from build123d import *

# Parameters (mm, degrees)
SKETCH1_W               = 6
SKETCH1_H               = 15
SKETCH1_W_2             = 8
SKETCH1_H_2             = 28.7
BOSS_EXTRUDE1_DEPTH     = 9
SKETCH2_R               = 2.65
CUT_EXTRUDE1_DEPTH      = 34.176648414
SKETCH5_W               = 10
SKETCH5_H               = 5.3
BOSS_EXTRUDE4_DEPTH     = 5
SKETCH6_W               = 12
SKETCH6_H               = 5.3
BOSS_EXTRUDE5_DEPTH     = 2
SKETCH7_W               = 14
SKETCH7_H               = 6.2
CUT_EXTRUDE2_DEPTH      = 1.2
SKETCH8_R               = 1.45
CUT_EXTRUDE3_DEPTH      = 8
CUT_EXTRUDE4_DEPTH      = 36.716802768
CUT_EXTRUDE4_DEPTH_BACK = 36.716802768
SKETCH9_R               = 1.75
FILLET1_R               = 5
FILLET2_R               = 6
FILLET3_R               = 3


# Some blends are built 0.0001 mm under size
with BuildPart() as part:
    # Sketch1 → Boss-Extrude1 (new, symmetric)
    with BuildSketch(Plane.XY):
        with Locations((11, -7.5)):
            Rectangle(SKETCH1_W, SKETCH1_H)
        with Locations((4, -14.35)):
            Rectangle(SKETCH1_W_2, SKETCH1_H_2)
    extrude(amount=BOSS_EXTRUDE1_DEPTH, both=True)

    # Sketch2 → Cut-Extrude1 (cut, through all)
    with BuildSketch(Plane(origin=(14, 0, 0), x_dir=(0, 0, -1), z_dir=(1, 0, 0))):
        with Locations(Location((5, -4.2, 0), (0, 0, 90))):
            Circle(SKETCH2_R)
        with Locations(Location((-5, -4.2, 0), (0, 0, 90))):
            Circle(SKETCH2_R)
    extrude(amount=-CUT_EXTRUDE1_DEPTH, mode=Mode.SUBTRACT)

    # Sketch5 → Boss-Extrude4 (add)
    with BuildSketch(Plane.XY.offset(9)):
        with Locations((5, -4.2)):
            Rectangle(SKETCH5_W, SKETCH5_H)
    boss_extrude4 = extrude(amount=BOSS_EXTRUDE4_DEPTH)

    # Sketch6 → Boss-Extrude5 (add)
    with BuildSketch(Plane.XY.offset(14)):
        with Locations((6, -4.2)):
            Rectangle(SKETCH6_W, SKETCH6_H)
    boss_extrude5 = extrude(amount=BOSS_EXTRUDE5_DEPTH)

    # Mirror2: Boss-Extrude4, Boss-Extrude5 across plane
    add(boss_extrude4.mirror(Plane.XY))
    add(boss_extrude5.mirror(Plane.XY))

    # Sketch7 → Cut-Extrude2 (cut)
    with BuildSketch(Plane(origin=(0, 0, 0), x_dir=(1, 0, 0), z_dir=(0, 1, 0))):
        with Locations((7, 0)):
            Rectangle(SKETCH7_W, SKETCH7_H)
    extrude(amount=-CUT_EXTRUDE2_DEPTH, mode=Mode.SUBTRACT)

    # Sketch8 → Cut-Extrude3 (cut)
    with BuildSketch(Plane(origin=(0, -1.2, 0), x_dir=(1, 0, 0), z_dir=(0, 1, 0))):
        with Locations(Location((7, 0, 0), (0, 0, 270))):
            Circle(SKETCH8_R)
    extrude(amount=-CUT_EXTRUDE3_DEPTH, mode=Mode.SUBTRACT)

    # Sketch9 → Cut-Extrude4 (cut, two sides: drawn at the far end of the back side and taken through both)
    with BuildSketch(Plane.ZY.offset(-CUT_EXTRUDE4_DEPTH_BACK)):
        with Locations(Location((0, -18.7, 0), (0, 0, 90))):
            Circle(SKETCH9_R)
    extrude(amount=CUT_EXTRUDE4_DEPTH + CUT_EXTRUDE4_DEPTH_BACK, mode=Mode.SUBTRACT)

    # Fillet1
    fillet1_edges = [part.edges().sort_by_distance(p)[0] for p in [
        (8, -28.7, 0),
    ]]
    fillet(fillet1_edges, radius=FILLET1_R)

    # Fillet2
    fillet2_edges = [part.edges().sort_by_distance(p)[0] for p in [
        (14, -15, 0),
    ]]
    fillet(fillet2_edges, radius=FILLET2_R - 0.0001)  # a hair under: the kernel refuses the full size

    # Fillet3
    # the kernel refuses this fillet: 3 mm, written as the material it adds along each edge
    with BuildSketch(Plane(origin=(10, -6.85, 9), x_dir=(0, -1, 0), z_dir=(-1, 0, 0))) as fillet3_piece_1:
        with BuildLine():
            CenterArc((FILLET3_R, FILLET3_R), FILLET3_R, 180, 90)
            Line((0, FILLET3_R), (-FILLET3_R * 0.02, FILLET3_R))
            Line((-FILLET3_R * 0.02, FILLET3_R), (-FILLET3_R * 0.02, -FILLET3_R * 0.02))
            Line((-FILLET3_R * 0.02, -FILLET3_R * 0.02), (FILLET3_R, -FILLET3_R * 0.02))
            Line((FILLET3_R, -FILLET3_R * 0.02), (FILLET3_R, 0))
        make_face()
    extrude(amount=10)
    with BuildSketch(Plane(origin=(0, -1.55, 9), x_dir=(0, 1, 0), z_dir=(1, 0, 0))) as fillet3_piece_2:
        with BuildLine():
            CenterArc((3, 2.626309197), FILLET3_R, 180, 61.09666546)
            Line((0, 2.626309197), (-0.06, 2.626309197))
            Line((-0.06, 2.626309197), (-0.06, 0))
            Line((-0.06, 0), (0, -0.06))
            ThreePointArc((0, -0.06), (0.775, -0.06), (1.521, -0.052526184))
            Line((1.521, -0.052526184), (1.55, 0))
        make_face()
    extrude(amount=10)
    with BuildSketch(Plane(origin=(10, -6.85, -9), x_dir=(0, -1, 0), z_dir=(-1, 0, 0))) as fillet3_piece_3:
        with BuildLine():
            CenterArc((FILLET3_R, -FILLET3_R), FILLET3_R, 90, 90)
            Line((0, -FILLET3_R), (-FILLET3_R * 0.02, -FILLET3_R))
            Line((-FILLET3_R * 0.02, -FILLET3_R), (-FILLET3_R * 0.02, FILLET3_R * 0.02))
            Line((-FILLET3_R * 0.02, FILLET3_R * 0.02), (FILLET3_R, FILLET3_R * 0.02))
            Line((FILLET3_R, FILLET3_R * 0.02), (FILLET3_R, 0))
        make_face()
    extrude(amount=10)
    with BuildSketch(Plane(origin=(0, -1.55, -9), x_dir=(0, 1, 0), z_dir=(1, 0, 0))) as fillet3_piece_4:
        with BuildLine():
            CenterArc((3, -2.626309197), FILLET3_R, 118.90333454, 61.09666546)
            Line((0, -2.626309197), (-0.06, -2.626309197))
            Line((-0.06, -2.626309197), (-0.06, 0))
            Line((-0.06, 0), (0, 0.06))
            ThreePointArc((0, 0.06), (0.775, 0.06), (1.521, 0.052526184))
            Line((1.521, 0.052526184), (1.55, 0))
        make_face()
    extrude(amount=10)


solid = part.part
Geometry: final body of the model. Coordinates: model frame, mm. A direction names the side the tool comes from. Give positions to 0.01 mm unless a question says otherwise; leave off trailing zeros. Write each loop counter-clockwise with the first axis right and the second up, starting at its lowest first coordinate (ties: lowest second). Pieces come first, ordered by that corner, then holes. Notation, with made-up numbers: M -30,39.5 L -11,39.5 A29 cw -11,72.5 Z; hole C 85,22 d8. An arc over 180 degrees is marked long. Answer in a Markdown table with one row per item. Add a question column.
(1) First-contact query: pin 1 (0.9 mm diameter, centred on x = 7, z = 0, fed in from +Y); pin 2 (5 mm diameter, centred on x = 5, y = -20.5, fed in from -Z); pin 3 (2 mm diameter, centred on x = 9, z = 11.5, fed in from -Y). Flat tips, straight axial feed; report the tip coordinate or a pass-through.
(2) Mould query, pull axis Z, two halves, no side actions, for faces 4 (the cylindrical face through (5.07, -7.75, -9.86)), 5 (the cylindrical face through (7.098, -6.303, -6.612)), 6 (the flat face through (7, -9.2, 0)), 7 (the flat face through (6, -6.85, 14)). Classes: +Z half, -Z half, draft (parallel to the pull), parting line (faces both ways), or undercut.
(3) Reachability of faces 1 (the flat face through (12, -4, 15)), 2 (the flat face through (6, -6.85, -14)), 3 (the flat face through (11, -4, -14)) from +Z, -Z, +X, -X, +Y, -Y: full face, straight path, thin tool, end or side. Return the list, or none.
(4) Ray query, line 1 (Z direction, x = 8.75, y = -4.2); line 2 (Z direction, x = 10.75, y = -4.2); line 3 (X direction, y = -6, z = 0). Return the intervals inside material, ascending.
(5) Section D-D on x = 7. Return loops of the section in (y, z), and give its area (3 significant figures).
(6) Section A-A on y = -4.2. Return loops of the section in (x, z), and give its area (3 significant figures).
(7) Section C-C on y = -18.7. Return loops of the section in (x, z), and give its area (3 significant figures).
Result set:
| question | item | result |
|---|---|---|
| 1 | pin 1 | stops at y = -9.2 |
| 1 | pin 2 | stops at z = -9 |
| 1 | pin 3 | stops at y = -7.25 |
| 2 | face 4 | -Z half |
| 2 | face 5 | undercut |
| 2 | face 6 | undercut |
| 2 | face 7 | draft |
| 3 | face 1 | +Z, +X, +Y, -Y |
| 3 | face 2 | -Z, +X, -X, -Y |
| 3 | face 3 | +X, +Y, -Y |
| 4 | line 1 | z = -16 to -7.65, -2.35 to 2.35, 7.65 to 16 |
| 4 | line 2 | z = -16 to -14, -9 to -7.65, -2.35 to 2.35, 7.65 to 9, 14 to 16 |
| 4 | line 3 | x = 0 to 5.55, 8.45 to 14 |
| 5 | outline | M -26.7,-9 L -9.85,-9 A3 cw -6.85,-12 L -6.85,-16 L -1.55,-16 L -1.55,-11.63 A3 cw 0,-9 L 0,-3.1 L -1.2,-3.1 L -1.2,-1.45 L -9.2,-1.45 L -9.2,1.45 L -1.2,1.45 L -1.2,3.1 L 0,3.1 L 0,9 A3 cw -1.55,11.63 L -1.55,16 L -6.85,16 L -6.85,12 A3 cw -9.85,9 L -26.7,9 Z; hole C -18.7,0 d3.5; hole C -4.2,-5 d5.3; hole C -4.2,5 d5.3 |
| 5 | area | 477 mm^2 |
| 6 | outline | M 0,-16 L 12,-16 L 12,-14 L 10,-14 L 10,-9 L 14,-9 L 14,-7.65 L 0,-7.65 Z; M 0,-2.35 L 14,-2.35 L 14,2.35 L 0,2.35 Z; M 0,7.65 L 14,7.65 L 14,9 L 10,9 L 10,14 L 12,14 L 12,16 L 0,16 Z; hole C 7,0 d2.9 |
| 6 | area | 245 mm^2 |
| 7 | outline | M 0,-9 L 8,-9 L 8,-1.75 L 0,-1.75 Z; M 0,1.75 L 8,1.75 L 8,9 L 0,9 Z |
| 7 | area | 116 mm^2 |
